The drawing under review shows one solid part. Ordinate dimensions are in mm from its lowest x, y, z. A direction names the side the tool comes from. Round coordinates to 2 decimals unless told otherwise and drop trailing zeros. Order: outer loops, then holes, each group sorted by start corner. A loop starts at its lowest first (then second) coordinate and runs counter-clockwise, first axis right, second up. Notation, with made-up numbers: M -3.5,-0.5 L 4.5,-0.5 A17 cw 4.5,11.5 Z; hole C 29.5,8.5 d8. An arc over 180 degrees is marked long. Answer in a Markdown table with one row per item. Add a question column.
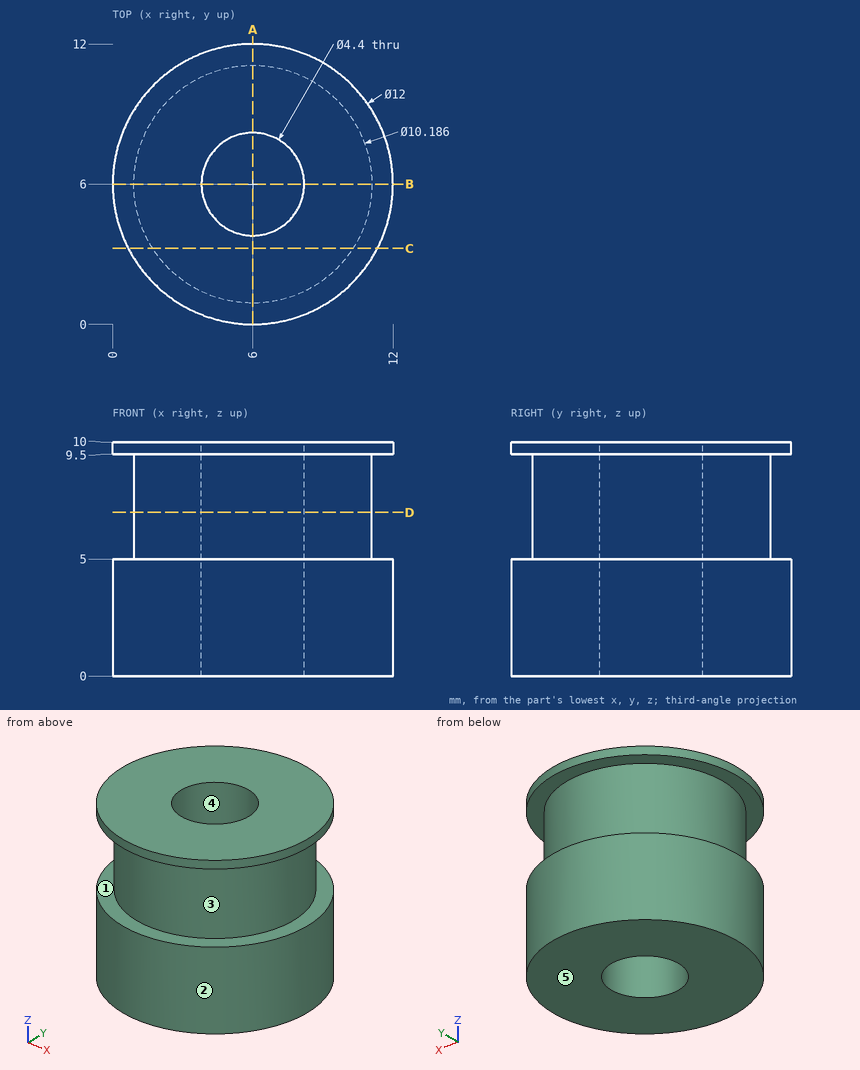
1. Consider section D-D on z = 7. Write out the cut boundary in (x, y).
2. Clearance check with flat-ended pins moving along their axes: pin 1 Ø1.5 at (y, z) = (5.5, 8.5) entering from +X; pin 2 Ø2.5 at (x, y) = (6, 6) entering from -Z. State where each tip first meets the part, or that it passes through.
3. Consider section A-A on x = 6. Write out the cut boundary in (y, z).
4. The part is to be moulded in two halves that separate along X. For the marked faces 3, 4 and 5, say which applies: pulls with the +X half, pulls with the -X half, needs draft (parallel to the pull), parting line crosses it, or undercut.
5. To check wall thickness, follow probe 1 along Y at (x, z) = (6, 3.25); probe 2 along Y at (x, z) = (6, 7.25); probe 3 along X at (y, z) = (7, 4.25). State the ranges of each line that lie inside material, in increasing order. Write a range as [from, to].
6. For the marked faces 1 and 2, list the 3-axis set-ups (+Z, -Z, +X, -X, +Y, -Y) from which the entire face can be reached by the end or side of a thin tool; tool diameter is ignored.
7. Consider section C-C on y = 3.25. Write out the cut boundary in (x, z), plus the area to 3 significant figures.
Solved:
| question | item | result |
|---|---|---|
| 1 | outline | C 6,6 d10.19; hole C 6,6 d4.4 |
| 2 | pin 1 | stops at x = 11.09 |
| 2 | pin 2 | passes through |
| 3 | outline | M 0,0 L 3.8,0 L 3.8,10 L 0,10 L 0,9.5 L 0.91,9.5 L 0.91,5 L 0,5 Z; M 8.2,0 L 12,0 L 12,5 L 11.09,5 L 11.09,9.5 L 12,9.5 L 12,10 L 8.2,10 Z |
| 4 | face 3 | parting line crosses it |
| 4 | face 4 | undercut |
| 4 | face 5 | needs draft |
| 5 | probe 1 | y = [0, 3.8], [8.2, 12] |
| 5 | probe 2 | y = [0.91, 3.8], [8.2, 11.09] |
| 5 | probe 3 | x = [0.08, 4.04], [7.96, 11.92] |
| 6 | face 1 | none |
| 6 | face 2 | +Z, -Z |
| 7 | outline | M 0.67,0 L 11.33,0 L 11.33,5 L 10.29,5 L 10.29,9.5 L 11.33,9.5 L 11.33,10 L 0.67,10 L 0.67,9.5 L 1.71,9.5 L 1.71,5 L 0.67,5 Z |
| 7 | area | 97.2 mm^2 |
